The model under review builds one solid part; all positions refer to its coordinate system, in mm. A direction names the side the tool comes from. Round coordinates to 2 decimals unless told otherwise and drop trailing zeros. Order: outer loops, then holes, each group sorted by start corner. A loop starts at its lowest first (then second) coordinate and runs counter-clockwise, first axis right, second up.
from build123d import *

# Parameters (mm, degrees)
BOSS_EXTRU_2_DEPTH           = 235
ESQUISSE2_R                  = 44.45
ENL_V_MAT_EXTRU_1_DEPTH      = 78
ESQUISSE3_R                  = 28.575
ENL_V_MAT_EXTRU_2_DEPTH      = 190
ENL_V_MAT_EXTRU_3_DEPTH      = 13
BOSS_EXTRU_3_DEPTH           = 111
ESQUISSE10_W                 = 33
ESQUISSE10_H                 = 39.549429839
ENL_V_MAT_EXTRU_5_DEPTH      = 19
ENL_V_MAT_EXTRU_6_REACH      = 313.068
ENL_V_MAT_EXTRU_6_END_RADIUS = 28.575
ESQUISSE11_W                 = 19
ESQUISSE11_H                 = 33


with BuildPart() as part:
    # Esquisse1 → Boss.-Extru.2 (new body)
    with BuildSketch(Plane.XY):
        with BuildLine():
            Line((0, 0), (-13, 0))
            Line((-13, 0), (-86, 42.146569651))
            Line((-86, 42.146569651), (-86, 85.999071056))
            ThreePointArc((-86, 85.999071056), (-60.811511616, 146.810854752), (0, 172))
            Line((0, 172), (0, 0))
        make_face()
    extrude(amount=BOSS_EXTRU_2_DEPTH)

    # Esquisse2 → Enlèv. mat.-Extru.1 (cut)
    with BuildSketch(Plane.XY.offset(235)):
        with Locations((0, 86)):
            Circle(ESQUISSE2_R)
    extrude(amount=-ENL_V_MAT_EXTRU_1_DEPTH, mode=Mode.SUBTRACT)

    # Esquisse3 → Enlèv. mat.-Extru.2 (cut)
    with BuildSketch(Plane.XY.offset(157)):
        with Locations((0, 86)):
            Circle(ESQUISSE3_R)
    extrude(amount=-ENL_V_MAT_EXTRU_2_DEPTH, mode=Mode.SUBTRACT)

    # Esquisse4 → Enlèv. mat.-Extru.3 (cut)
    with BuildSketch(Plane(origin=(0, 0, 0), x_dir=(0, 0, -1), z_dir=(1, 0, 0))):
        with BuildLine():
            Line((0, 17.7125), (-110, 17.7125))
            ThreePointArc((-110, 17.7125), (-121, 28.7125), (-110, 39.7125))
            Line((-110, 39.7125), (0, 39.7125))
            ThreePointArc((0, 39.7125), (11, 28.7125), (0, 17.7125))
        make_face()
    extrude(amount=-ENL_V_MAT_EXTRU_3_DEPTH, mode=Mode.SUBTRACT)

    # Esquisse7 → Boss.-Extru.3 (add)
    with BuildSketch(Plane.XY.offset(157)):
        with BuildLine():
            Line((-34.329616244, 164.850982549), (-14.946427951, 149.707176139))
            Line((-14.946427951, 149.707176139), (-40.188548439, 117.398735242))
            Line((-40.188548439, 117.398735242), (-65.430668927, 85.090294344))
            Line((-65.430668927, 85.090294344), (-84.81385722, 100.234100753))
            ThreePointArc((-84.81385722, 100.234100753), (-67.768924815, 138.946886878), (-34.329616244, 164.850982549))
        make_face()
    extrude(amount=BOSS_EXTRU_3_DEPTH)

    # Esquisse10 → Enlèv. mat.-Extru.5 (cut)
    with BuildSketch(Plane(origin=(0, 0, 0), x_dir=(0, 0, -1), z_dir=(1, 0, 0))):
        with Locations((-54.5, 152.22528508)):
            Rectangle(ESQUISSE10_W, ESQUISSE10_H)
    extrude(amount=-ENL_V_MAT_EXTRU_5_DEPTH, mode=Mode.SUBTRACT)

    # Enlèv. mat.-Extru.6: up to this cylinder (the profile starts outside it)
    enl_v_mat_extru_6_end = Plane(origin=(0, 86, 54.5), z_dir=(0, 0, 1)) * Cylinder(ENL_V_MAT_EXTRU_6_END_RADIUS, 684.286, mode=Mode.PRIVATE)
    # Esquisse11 → Enlèv. mat.-Extru.6 (cut, up to the surface)
    with BuildSketch(Plane(origin=(0, 132.450570161, 0), x_dir=(1, 0, 0), z_dir=(0, 1, 0)), mode=Mode.PRIVATE) as enl_v_mat_extru_6_sk1:
        with Locations((-9.5, -54.5)):
            Rectangle(ESQUISSE11_W, ESQUISSE11_H)
    enl_v_mat_extru_6_tool1 = extrude(enl_v_mat_extru_6_sk1.sketch, amount=-ENL_V_MAT_EXTRU_6_REACH, mode=Mode.PRIVATE) - enl_v_mat_extru_6_end
    add(enl_v_mat_extru_6_tool1.solids().sort_by_distance((-9.5, 132.45057, 54.5))[0], mode=Mode.SUBTRACT)


solid = part.part
(1) Clearance check with flat-ended pins moving along their axes: P1, Ø1.5, axis at x = -40, z = 221.5, coming from the -Y side; P2, Ø9.5, axis at x = -7, y = 139.5, coming from the +Z side; P3, Ø11, axis at y = 31, z = 60.5, coming from the +X side. State where each tip first meets the part, or that it passes through.
(2) Tool access review of faces 4 (the flat face through (-74.99, 92.56, 251.27)), 5 (the flat face through (-9, 139, 71)), 6 (the cylindrical face through (-6.409, 28.471, 120.997)), 7 (the flat face through (0, 144, 152)): name each direction out of +Z, -Z, +X, -X, +Y, -Y from which nothing blocks a thin tool from reaching the whole face with its end or side.
(3) The part is to be moulded in two halves that separate along Y. For faces 1 (the flat face through (-24.774, 157.385, 251.269)), 2 (the flat face through (-32, 87, 157)), 3 (the flat face through (-6, 0, 116)), say which applies: pulls with the +Y half, pulls with the -Y half, needs draft (parallel to the pull), parting line crosses it, or undercut.
(4) To check wall thickness, follow L1, parallel to Y at x = -8, z = 34; L2, parallel to Z at x = -23.5, y = 45; L3, parallel to Y at x = -17.5, z = 123. State the ranges of each line that lie inside material, in increasing order.
(5) We need section B-B (y = 67). Give the boundary of the cut face in (x, z), and give its area (3 significant figures).
(6) We need section C-C (x = -72). Give the boundary of the cut face in (y, z), and give its area (3 significant figures).
Verdict:
1. P1: stops at y = 15.16
1. P2: stops at z = 235
1. P3: stops at x = -13
2. face 4: +Z, -X, -Y
2. face 5: +X, +Y
2. face 6: -Z, +X
2. face 7: +Z, -Z, +X, +Y, -Y
3. face 1: pulls with the +Y half
3. face 2: undercut
3. face 3: pulls with the -Y half
4. L1: y = 0 to 17.71, 39.71 to 58.57, 113.43 to 171.63
4. L2: z = 0 to 235
4. L3: y = 2.6 to 63.41, 108.59 to 170.2
5. outline: (-86, 0) - (-21.34, 0) - (-21.34, 157) - (-40.18, 157) - (-40.18, 235) - (-86, 235) - close
5. area: 13,700 mm2
6. outline: (34.06, 0) - (133.03, 0) - (133.03, 268) - (90.22, 268) - (90.22, 235) - (34.06, 235) - close
6. area: 24,700 mm2
